Check sheet for the drawn part. Datum: minimum x, y, z corner. Units: mm. A direction names the side the tool comes from. Give positions to 0.01 mm unless a question says otherwise; leave off trailing zeros. Write each loop counter-clockwise with the first axis right and the second up, starting at its lowest first coordinate (ties: lowest second). Pieces come first, ordered by that corner, then holes. Notation, with made-up numbers: M 89,35.25 L 98,35.25 A7 ccw 98,44.25 Z; hole C 57.25,-4 d4. An arc over 180 degrees is marked long. Write item = value, one per line. Start each with the question number.
1) Sectioned sample at A-A, the plane x = 300. Record the cut outline in (y, z).
2) Sectioned sample at B-B, the plane z = 75. Record the cut outline in (x, y), then the cut area to 4 significant figures.
3) Gauge pin test, flat ends, axial feed: pin 1 (9 mm diameter, centred on x = 365, y = 25, fed in from -Z); pin 2 (9 mm diameter, centred on x = 25, y = 25, fed in from -Z); pin 3 (11 mm diameter, centred on x = 365.5, y = 27, fed in from +Z). Record the tip position at first contact, or that the pin passes through.
4) Sectioned sample at D-D, the plane x = 25. Record the cut outline in (y, z), then the cut area to 3 significant figures.
5) Scan lines: L1, parallel to Z at x = 300, y = 12; L2, parallel to X at y = 25, z = 10; L3, parallel to Z at x = 75, y = 25.5. Record each from-to range of solid material in increasing order.
6) Set-up check for the marked faces 1 and 2: record each of +Z, -Z, +X, -X, +Y, -Y from which the full face is reachable in a straight line by a thin tool's end or side.
7) Sectioned sample at C-C, the plane y = 45. Record the cut outline in (x, z), then the cut area to 3 significant figures.
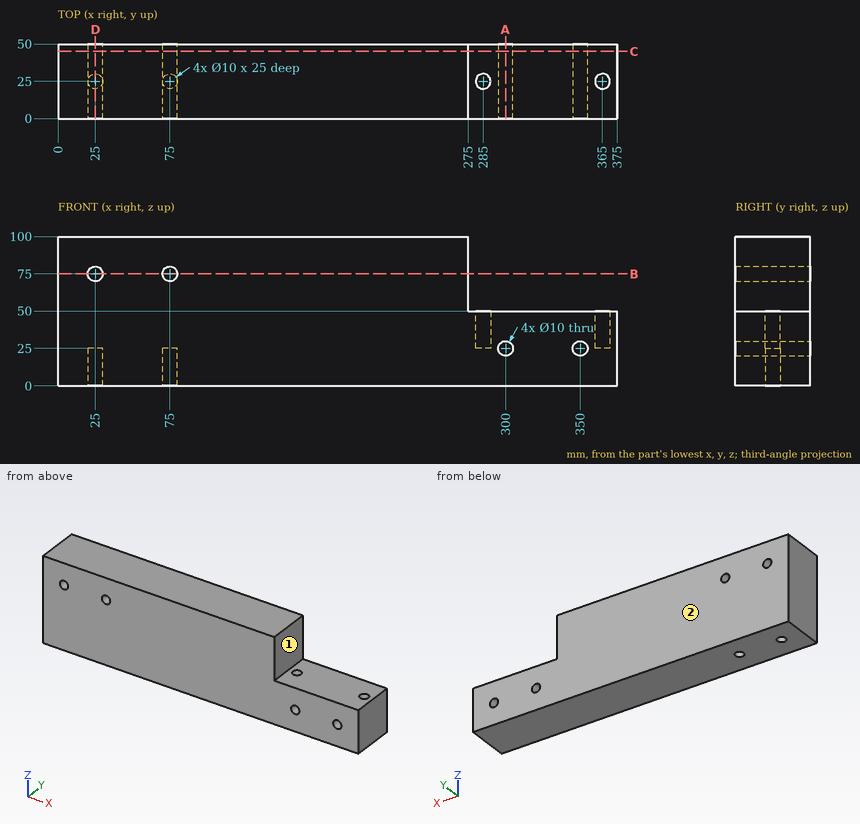
Data:
q1.outline = M 0,0 L 50,0 L 50,20 L 0,20 Z; M 0,30 L 50,30 L 50,50 L 0,50 Z
q2.outline = M 0,0 L 20,0 L 20,50 L 0,50 Z; M 30,0 L 70,0 L 70,50 L 30,50 Z; M 80,0 L 275,0 L 275,50 L 80,50 Z
q2.area = 12,750 mm2
q3.pin_1 = 0
q3.pin_2 = 25
q3.pin_3 = 50
q4.outline = M 0,0 L 20,0 L 20,25 L 30,25 L 30,0 L 50,0 L 50,70 L 0,70 Z; M 0,80 L 50,80 L 50,100 L 0,100 Z
q4.area = 4,250 mm2
q5.L1 = 0 to 20, 30 to 50
q5.L2 = 0 to 20, 30 to 70, 80 to 375
q5.L3 = 25 to 70, 80 to 100
q6.face_1 = +Z, +X, +Y, -Y
q6.face_2 = +Z, -Z, +X, -X, +Y
q7.outline = M 0,0 L 375,0 L 375,50 L 275,50 L 275,100 L 0,100 Z; hole C 25,75 d10; hole C 75,75 d10; hole C 300,25 d10; hole C 350,25 d10
q7.area = 32,200 mm2
